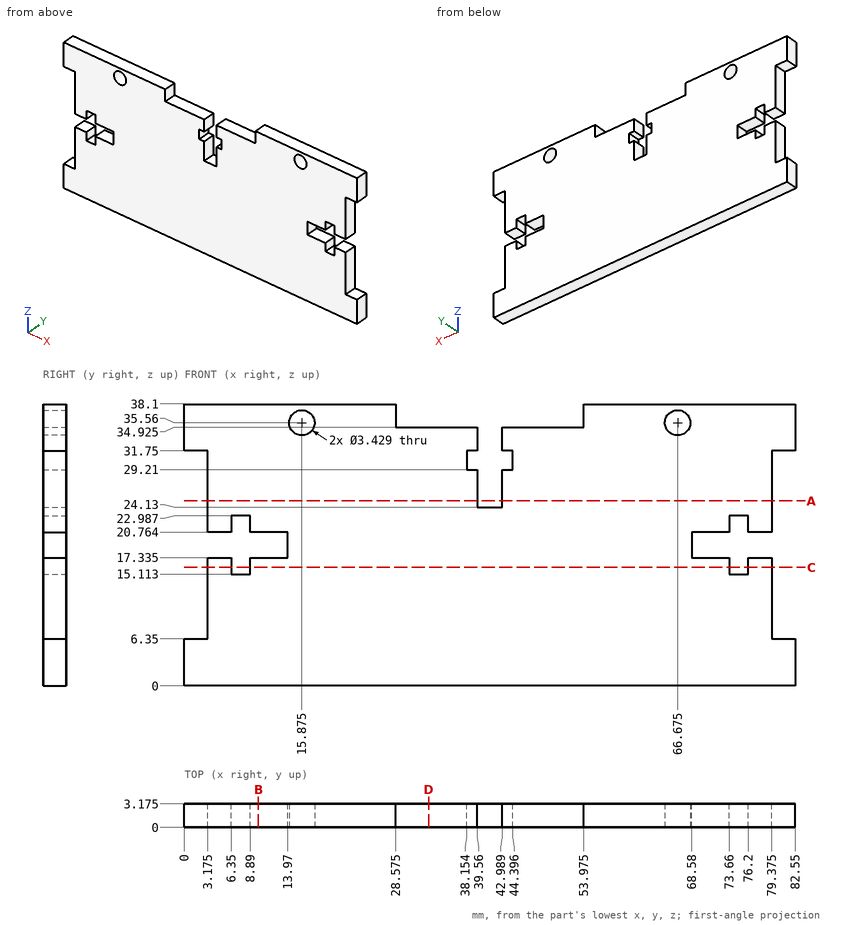
Verification items for this drawing (mm, ordinates from the low corner). Coordinates: 2 decimals unless noted, no trailing zeros. Order: outer loops, then holes, each group sorted by start corner. A loop starts at its lowest first (then second) coordinate and runs counter-clockwise, first axis right, second up. Notation, with made-up numbers: M 85,-26.5 L 141,-26.5 A14 cw 141,-15.5 Z; hole C 77,-6.75 d11. An arc over 180 degrees is marked long. Write each question's results on one line, items separated by ' | '.
1) Section check A-A on z = 25. Record the cut outline in (x, y) (1 decimal), plus the area to 3 significant figures.
Solved:
outline: M 3.2,0 L 39.6,0 L 39.6,3.2 L 3.2,3.2 Z; M 43,0 L 79.4,0 L 79.4,3.2 L 43,3.2 Z | area: 231 mm²
2) Section check C-C on z = 16. Give the number of separate pieces and of enclosed holes in the cut face, plus the area to 3 significant figures.
Solved:
separate pieces: 3 | enclosed holes: 0 | area: 226 mm²
3) Gauge pin test, flat ends, axial feed: pin 1 Ø1 at (y, z) = (1, 10) entering from -X (1 decimal); pin 2 Ø0.7 at (y, z) = (2.5, 16) entering from +X (1 decimal). Record the tip position at first contact, or that the pin passes through.
Solved:
pin 1: stops at x = 3.2 | pin 2: stops at x = 79.4
4) Scan lines: line 1 along Z through (x, y) = (11.5, 2.25) (1 decimal); line 2 along X through (y, z) = (1.9, 25.5) (1 decimal); line 3 along Z through (x, y) = (51.5, 0.25) (1 decimal). Record each from-to range of solid material in increasing order. Write a range as [from, to].
Solved:
line 1: z = [0, 17.3], [20.8, 38.1] | line 2: x = [3.2, 39.6], [43, 79.4] | line 3: z = [0, 34.9]
5) Section check B-B on x = 10. Record the cut outline in (y, z) (1 decimal), plus the area to 3 significant figures.
Solved:
outline: M 0,0 L 3.2,0 L 3.2,17.3 L 0,17.3 Z; M 0,20.8 L 3.2,20.8 L 3.2,38.1 L 0,38.1 Z | area: 110 mm²
6) Section check D-D on x = 33. Record the cut outline in (y, z) (1 decimal), plus the area to 3 significant figures.
Solved:
outline: M 0,0 L 3.2,0 L 3.2,34.9 L 0,34.9 Z | area: 111 mm²
